from build123d import *

# Parameters (mm, degrees)
SKETCH1_R           = 4.75
BOSS_EXTRUDE1_DEPTH = 0.0001
BOSS_EXTRUDE2_START = 105
SKETCH4_R           = 4.75
BOSS_EXTRUDE2_DEPTH = 105
CUT_EXTRUDE3_DEPTH  = 4
SKETCH6_R           = 4.75
CUT_EXTRUDE4_DEPTH  = 5


with BuildPart() as part:
    # Sketch1 → Boss-Extrude1 (new body)
    with BuildSketch(Plane.XY):
        Circle(SKETCH1_R)
    extrude(amount=BOSS_EXTRUDE1_DEPTH)

    # Sketch4 → Boss-Extrude2 (add)
    with BuildSketch(Plane(origin=(0, 0, 0), x_dir=(-1, 0, 0), z_dir=(0, 0, -1)).offset(BOSS_EXTRUDE2_START)):
        Circle(SKETCH4_R)
    extrude(amount=-BOSS_EXTRUDE2_DEPTH)

    # Sketch5 → Cut-Extrude3 (cut)
    with BuildSketch(Plane(origin=(0, 4.75, 0), x_dir=(1, 0, 0), z_dir=(0, 1, 0))):
        with BuildLine():
            Line((-2, 10), (-2, 20))
            ThreePointArc((-2, 20), (0, 22), (2, 20))
            Line((2, 20), (2, 10))
            ThreePointArc((2, 10), (0, 8), (-2, 10))
        make_face()
        with BuildLine():
            Line((-2, 69.62), (-2, 74.62))
            ThreePointArc((-2, 74.62), (0, 76.62), (2, 74.62))
            Line((2, 74.62), (2, 69.62))
            ThreePointArc((2, 69.62), (0, 67.62), (-2, 69.62))
        make_face()
    extrude(amount=-CUT_EXTRUDE3_DEPTH, mode=Mode.SUBTRACT)

    # Sketch6 → Cut-Extrude4 (cut)
    with BuildSketch(Plane(origin=(0, 0, -105), x_dir=(-1, 0, 0), z_dir=(0, 0, -1))):
        Circle(SKETCH6_R)
    extrude(amount=-CUT_EXTRUDE4_DEPTH, mode=Mode.SUBTRACT)


solid = part.part
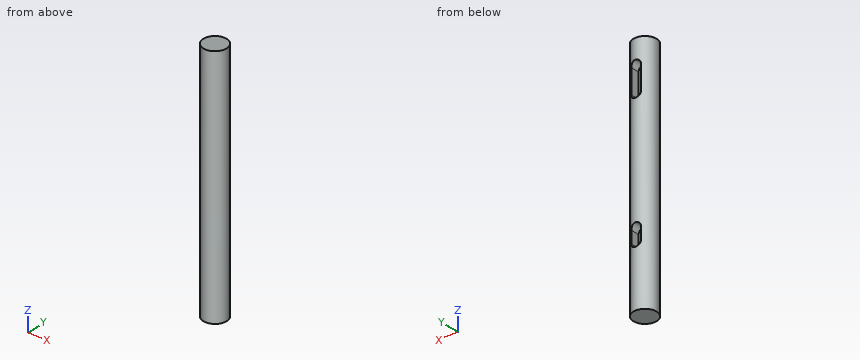
Check sheet for the modelled part. Datum: model origin and axes. Units: mm. Give positions to 0.01 mm unless a question says otherwise; leave off trailing zeros. Order: outer loops, then holes, each group sorted by start corner. A loop starts at its lowest first (then second) coordinate and runs counter-clockwise, first axis right, second up. Notation, with made-up numbers: (-33, 31) - (14, 31) arc R25 ccw to (14, 63) - close; hole circle Ø1 at (-31, -2). An arc over 180 degrees is marked (long way). Answer as CSV lines item,"result".
1. Scan lines: probe 1 along Z at (x, y) = (1, 2.25); probe 2 along Z at (x, y) = (-1.25, 1); probe 3 along X at (y, z) = (-0.25, -17.5). Record each from-to range of solid material in increasing order. Write a range as from..to.
Result sheet:
probe 1,"-100..-76.35, -67.89..-21.73, -8.27..0"
probe 2,"-100..-76.18, -68.06..-21.56, -8.44..0"
probe 3,"-4.74..4.74"
2. Section check D-D (y = -3). Record the boundary of the cut face in (x, z), then the cut area to 3 significant figures.
Result sheet:
outline,"(-3.68, -100) - (3.68, -100) - (3.68, 0) - (-3.68, 0) - close"
area,"737 mm²"
3. Section check A-A (x = 0). Record the boundary of the cut face in (y, z), then the cut area to 3 significant figures.
Result sheet:
outline,"(-4.75, -100) - (4.75, -100) - (4.75, -76.62) - (0.75, -76.62) - (0.75, -67.62) - (4.75, -67.62) - (4.75, -22) - (0.75, -22) - (0.75, -8) - (4.75, -8) - (4.75, 0) - (-4.75, 0) - close"
area,"858 mm²"
4. Section check B-B (y = 2). Record the boundary of the cut face in (x, z).
Result sheet:
outline,"(-4.31, -100) - (4.31, -100) - (4.31, 0) - (-4.31, 0) - close; hole (-2, -74.62) arc R2 ccw to (2, -74.62) - (2, -69.62) arc R2 ccw to (-2, -69.62) - close; hole (-2, -20) arc R2 ccw to (2, -20) - (2, -10) arc R2 ccw to (-2, -10) - close"
5. Section check C-C (z = -27.5). Record the boundary of the cut face in (x, y), then the cut area to 3 significant figures.
Result sheet:
outline,"circle Ø9.5 at (0, 0)"
area,"70.9 mm²"
6. Go/stop test with flat-tipped pins: P1, Ø3, axis at y = 3, z = -72, coming from the +X side; P2, Ø1.8, axis at y = 2.5, z = -73, coming from the -X side; P3, Ø3, axis at y = 2, z = -15.5, coming from the +X side. Record where each tip stops, or that it passes through.
Result sheet:
P1,"x = 4.51"
P2,"x = -4.47"
P3,"x = 4.72"
